```python
from build123d import *

# Parameters (mm, degrees)
SKETCH_3_W                  = 12
SKETCH_3_H                  = 3.426661337
SKETCH_3_W_2                = 4
SKETCH_3_H_2                = 2.458257046
CUT_EXTRUDE_1_DEPTH         = 5
CUT_EXTRUDE_1_DEPTH_BACK    = 5
HOLE_WIZARD_3_2_3_2_1_D     = 3.2
HOLE_WIZARD_3_2_3_2_1_DEPTH = 14
HOLE_WIZARD_3_2_3_2_1_TIP   = 0.96137699
CUT_EXTRUDE_2_REACH         = 8.5
SKETCH_6_R                  = 1.5


with BuildPart() as part:
    # Эскиз1 → Повернуть1 (revolve)
    with BuildSketch(Plane.XY):
        Polygon((0, 0), (0, 4), (34, 4), (34, 2), (45.5, 2), (46, 1.5), (46, 0), align=None)
    revolve(axis=Axis((0, 0, 0), (1, 0, 0)))

    # Эскиз3 → Вырез-Вытянуть1 (cut, two sides)
    with BuildSketch(Plane.XY) as cut_extrude_1_sk:
        with Locations((15.5, -4.213330669)):
            Rectangle(SKETCH_3_W, SKETCH_3_H)
        with Locations((11.5, 3.729128523)):
            Rectangle(SKETCH_3_W_2, SKETCH_3_H_2)
    extrude(amount=CUT_EXTRUDE_1_DEPTH, mode=Mode.SUBTRACT)
    extrude(cut_extrude_1_sk.sketch, amount=-CUT_EXTRUDE_1_DEPTH_BACK, mode=Mode.SUBTRACT)

    # Диаметр отверстия Ø3.2 (3.2)1
    with Locations(Plane.ZY):
        with Locations((0, 0)):
            Hole(HOLE_WIZARD_3_2_3_2_1_D / 2, depth=HOLE_WIZARD_3_2_3_2_1_DEPTH)
            with Locations((0, 0, -(HOLE_WIZARD_3_2_3_2_1_DEPTH + HOLE_WIZARD_3_2_3_2_1_TIP / 2))):  # 118° drill point
                Cone(0, HOLE_WIZARD_3_2_3_2_1_D / 2, HOLE_WIZARD_3_2_3_2_1_TIP, mode=Mode.SUBTRACT)

    # Эскиз6 → Вырез-Вытянуть2 (cut, up to next)
    with BuildSketch(Plane(origin=(0, 2.5, 0), x_dir=(1, 0, 0), z_dir=(0, 1, 0)), mode=Mode.PRIVATE) as cut_extrude_2_sk1:
        with Locations((11.5, 0)):
            Circle(SKETCH_6_R)
    cut_extrude_2_tool1 = extrude(cut_extrude_2_sk1.sketch, amount=-CUT_EXTRUDE_2_REACH, mode=Mode.PRIVATE) & part.part
    add(cut_extrude_2_tool1.solids().sort_by_distance((11.5, 2.5, 0))[0], mode=Mode.SUBTRACT)


solid = part.part
```
Read the model definition and answer for the solid it produces. Units are mm, in the model's axes. A direction names the side the tool comes from. Give positions to 0.01 mm unless a question says otherwise; leave off trailing zeros. Loops run counter-clockwise (first coordinate to the right, second up) from the corner with the lowest first, then second, coordinate; pieces in that order, holes last.
Item 1: The part is cut by section C-C (y = 3). Write down the section's boundary in (x, z).
Item 2: For faces 1 (the flat face through (10, 2.5, -1)), 2 (the cylindrical face through (12.19, 1.76, 1.33)), 3 (the flat face through (0, -2, 0)), 4 (the flat face through (21.5, -3, 0)), 5 (the flat face through (34, -2, -1)), determine the directions among +Z, -Z, +X, -X, +Y, -Y from which every point of the face is accessible in a straight line to the end or side of a thin tool.
Item 3: The part is cut by section D-D (x = 22). Write down the section's boundary in (y, z).
Item 4: The part is cut by section A-A (x = 11.5). Write down the section's boundary in (y, z), and give its area (3 significant figures).
Item 5: Find the intervals of material crossed by line 1 along Y through (x, z) = (7, 0); line 2 along X through (y, z) = (-2.75, 2.25), in increasing order.
Item 6: Each of these flat-tipped pins is pushed along its axis until it touches: pin 1 Ø1 at (x, z) = (16, -2.5) entering from +Y; pin 2 Ø1.2 at (y, z) = (3, 1.5) entering from +X; pin 3 Ø2 at (x, z) = (11, -1) entering from +Y. Where does it stop, or does it pass through?
Item 7: The mould has two halves that part along Z. Classify faces 6 (the cylindrical face through (17.238, 3.695, -1.532)), 7 (the cylindrical face through (7.1, -1.56, 0.35)), 8 (the flat face through (46, 0, 0)): released by +Z, released by -Z, zero draft, split by the parting line, or undercut.
Item 8: The part is cut by section B-B (z = -2.5). Write down the section's boundary in (x, y), and give its area (3 significant figures).
Taken from the geometry:
1. outline: (0, -2.65) - (9.5, -2.65) - (9.5, 2.65) - (0, 2.65) - close; (13.5, -2.65) - (34, -2.65) - (34, 2.65) - (13.5, 2.65) - close
2. face 1: +Z, -Z, +Y
2. face 2: +Y
2. face 3: +Z, -Z, -X, +Y, -Y
2. face 4: +Z, -Z, -Y
2. face 5: +X
3. outline: circle Ø8 at (0, 0)
4. outline: (-2.5, -3.12) arc R4 ccw to (2.5, -3.12) - (2.5, -1.5) - (0.56, -1.5) arc R1.6 cw (long way) to (0.56, 1.5) - (2.5, 1.5) - (2.5, 3.12) arc R4 ccw to (-2.5, 3.12) - close
4. area: 25.6 mm2
5. line 1: y = -4 to -1.6, 1.6 to 4
5. line 2: x = 0 to 9.5, 21.5 to 34
6. pin 1: stops at y = 3.46
6. pin 2: stops at x = 34
6. pin 3: stops at y = 2.5
7. face 6: split by the parting line
7. face 7: undercut
7. face 8: zero draft
8. outline: (0, -3.12) - (9.5, -3.12) - (9.5, -2.5) - (21.5, -2.5) - (21.5, -3.12) - (34, -3.12) - (34, 3.12) - (13.5, 3.12) - (13.5, 2.5) - (9.5, 2.5) - (9.5, 3.12) - (0, 3.12) - close
8. area: 202 mm2
